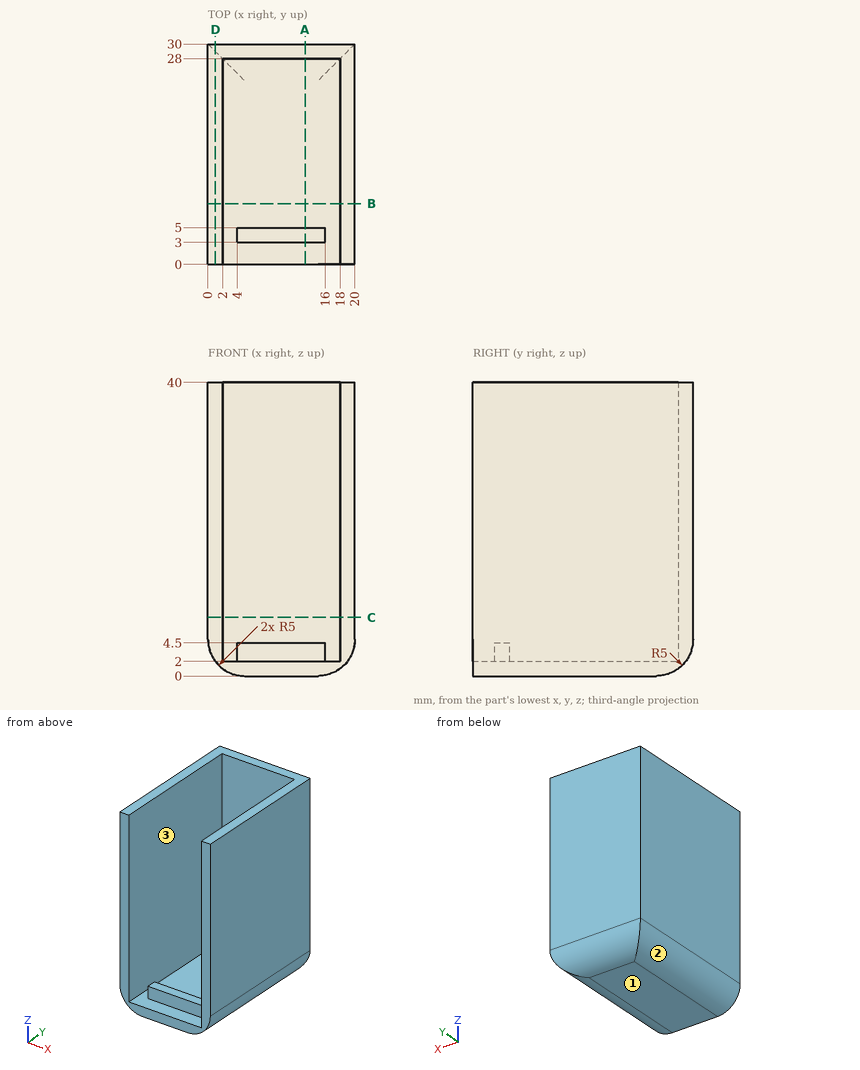
Geometry check sheet. Reference: drawing and pictorial views, mm from the part's lowest x, y, z. Coordinates: 2 decimals unless noted, no trailing zeros. Write each loop counter-clockwise with the first axis right and the second up, starting at its lowest first coordinate (ties: lowest second). Pieces come first, ordered by that corner, then holes. Notation, with made-up numbers: M -15,88.25 L 4,88.25 A16 ccw 4,97.25 Z; hole C -4.75,-34 d7. An arc over 180 degrees is marked long. Use one line per item in the form item = value.
Item 1: Sectioned sample at B-B, the plane y = 8.25. Record the cut outline in (x, z), and give its area (3 significant figures).
Answer below:
outline = M 0,5 A5 ccw 5,0 L 15,0 A5 ccw 20,5 L 20,40 L 18,40 L 18,2 L 2,2 L 2,40 L 0,40 Z
area = 181 mm^2
Item 2: Gauge pin test, flat ends, axial feed: pin 1 Ø10 at (x, z) = (12, 14.5) entering from -Y; pin 2 Ø0.8 at (x, z) = (11.5, 3.5) entering from -Y; pin 3 Ø8 at (x, y) = (9, 16.5) entering from +Z. Record the tip position at first contact, or that the pin passes through.
Answer below:
pin_1 = 28
pin_2 = 3
pin_3 = 2
Item 3: Sectioned sample at D-D, the plane x = 1. Record the cut outline in (y, z), and give its area (3 significant figures).
Answer below:
outline = M 0,2 L 29,2 A5 ccw 30,5 L 30,40 L 0,40 Z
area = 1,140 mm^2
Item 4: Material ranges on L1, parallel to X at y = 24.5, z = 35.5; L2, parallel to Y at x = 12.25, z = 21; L3, parallel to Z at x = 1, y = 28.25, recorded low to high. Write a range as from..to.
Answer below:
L1 = 0..2, 18..20
L2 = 28..30
L3 = 2..40
Item 5: Sectioned sample at C-C, the plane z = 8. Record the cut outline in (x, y).
Answer below:
outline = M 0,0 L 2,0 L 2,28 L 18,28 L 18,0 L 20,0 L 20,30 L 0,30 Z
Item 6: Release check for a two-part mould opening along X. For the marked faces 1, 2 and 3 record: pulls with the +X half, pulls with the -X half, needs draft (parallel to the pull), parting line crosses it, or undercut.
Answer below:
face_1 = needs draft
face_2 = pulls with the -X half
face_3 = undercut
Item 7: Sectioned sample at A-A, the plane x = 13.25. Record the cut outline in (y, z), and give its area (3 significant figures).
Answer below:
outline = M 0,0 L 25,0 A5 ccw 30,5 L 30,40 L 28,40 L 28,2 L 5,2 L 5,4.5 L 3,4.5 L 3,2 L 0,2 Z
area = 136 mm^2
